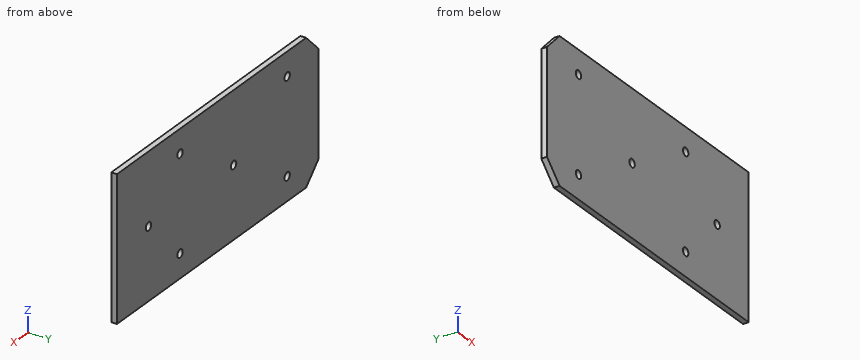
from build123d import *

# Parameters (mm, degrees)
F0_W     = 320
F0_H     = 150
F1_DEPTH = 6
F2_R     = 4.25
F3_DEPTH = 25
F4_SIZE  = 20


with BuildPart() as f1:
    # F0 (on Front) → F1 (new body)
    with BuildSketch(Plane.XZ):
        Rectangle(F0_W, F0_H)
    extrude(amount=F1_DEPTH)

    # F2 (on face) → F3 (cut)
    with BuildSketch(Plane(origin=(0, 0, 0), x_dir=(-1, 0, 0), z_dir=(0, 1, 0))):
        with Locations((-60, 50)):
            Circle(F2_R)
        with Locations((110, 50)):
            Circle(F2_R)
        with BuildLine():
            ThreePointArc((20.75, 0), (25, -4.25), (29.25, 0))
            Line((29.25, 0), (20.75, 0))
        make_face()
        with BuildLine():
            Line((20.75, 0), (29.25, 0))
            ThreePointArc((29.25, 0), (25, 4.25), (20.75, 0))
        make_face()
        with BuildLine():
            ThreePointArc((-114.25, 0), (-110, -4.25), (-105.75, 0))
            Line((-105.75, 0), (-114.25, 0))
        make_face()
        with BuildLine():
            Line((-114.25, 0), (-105.75, 0))
            ThreePointArc((-105.75, 0), (-110, 4.25), (-114.25, 0))
        make_face()
        with Locations((110, -50)):
            Circle(F2_R)
        with Locations((-60, -50)):
            Circle(F2_R)
    extrude(amount=-F3_DEPTH, mode=Mode.SUBTRACT)

    # F4
    f4_edges = [f1.edges().sort_by_distance(p)[0] for p in [
        (-160, -3, 75),
        (-160, -3, -75),
    ]]
    chamfer(f4_edges, length=F4_SIZE)


solid = f1.part
The model under review builds one solid part; all positions refer to its coordinate system, in mm. Give positions to 0.01 mm unless a question says otherwise; leave off trailing zeros. Write each loop counter-clockwise with the first axis right and the second up, starting at its lowest first coordinate (ties: lowest second). Pieces come first, ordered by that corner, then holes.
1. Wall thickness on L1, parallel to Z at x = -110, y = -3.35; L2, parallel to Z at x = -25, y = -3.5; L3, parallel to X at y = -4, z = -53: over which ranges is each line inside the solid? List them lowest first.
2. Add section B-B, the plane z = 0. Write out the cut boundary in (x, y), plus the area to 3 significant figures.
3. Add section C-C, the plane x = 60. Write out the cut boundary in (y, z), plus the area to 3 significant figures.
4. Add section D-D, the plane y = -1.5. Write out the cut boundary in (x, z), plus the area to 3 significant figures.
5. Add section A-A, the plane x = -25. Write out the cut boundary in (y, z), plus the area to 3 significant figures.
Worked answers:
1. L1: z = -75 to -54.25, -45.75 to 45.75, 54.25 to 75
1. L2: z = -75 to -4.25, 4.25 to 75
1. L3: x = -160 to -113.01, -106.99 to 56.99, 63.01 to 160
2. outline: (-160, -6) - (-29.25, -6) - (-29.25, 0) - (-160, 0) - close; (-20.75, -6) - (105.75, -6) - (105.75, 0) - (-20.75, 0) - close; (114.25, -6) - (160, -6) - (160, 0) - (114.25, 0) - close
2. area: 1,820 mm2
3. outline: (-6, -75) - (0, -75) - (0, -54.25) - (-6, -54.25) - close; (-6, -45.75) - (0, -45.75) - (0, 45.75) - (-6, 45.75) - close; (-6, 54.25) - (0, 54.25) - (0, 75) - (-6, 75) - close
3. area: 798 mm2
4. outline: (-160, -55) - (-140, -75) - (160, -75) - (160, 75) - (-140, 75) - (-160, 55) - close; hole circle Ø8.5 at (-110, -50); hole circle Ø8.5 at (-110, 50); hole circle Ø8.5 at (-25, 0); hole circle Ø8.5 at (60, -50); hole circle Ø8.5 at (60, 50); hole circle Ø8.5 at (110, 0)
4. area: 47,300 mm2
5. outline: (-6, -75) - (0, -75) - (0, -4.25) - (-6, -4.25) - close; (-6, 4.25) - (0, 4.25) - (0, 75) - (-6, 75) - close
5. area: 849 mm2
